The model under review builds one solid part; all positions refer to its coordinate system, in mm. Coordinates: 2 decimals unless noted, no trailing zeros. Write each loop counter-clockwise with the first axis right and the second up, starting at its lowest first coordinate (ties: lowest second). Pieces come first, ordered by that corner, then holes. Notation, with made-up numbers: (39.25, 48.5) - (47.25, 48.5) arc R14 cw to (47.25, 72.5) - close; hole circle Ø6 at (46.5, 87.5). An arc over 180 degrees is marked (long way). Put each result on its own line as item: value. Start each with the question number.
Item 1: To check wall thickness, follow L1, parallel to X at y = 3.5, z = -1; L2, parallel to X at y = 0.75, z = 25.5; L3, parallel to Z at x = 31, y = 3.5. State the ranges of each line that lie inside material, in increasing order. Write a range as [from, to].
Item 2: Consider section B-B on x = 0. Give the boundary of the cut face in (y, z), then the cut area to 3 significant figures.
Item 3: Consider section D-D on x = -56. Give the boundary of the cut face in (y, z).
Item 4: Consider section A-A on z = 0. Give the boundary of the cut face in (x, y), then the cut area to 3 significant figures.
Item 5: For pin 1 (1.9 mm diameter, centred on x = -60, y = 4.5, fed in from -Z); pin 2 (1.5 mm diameter, centred on y = 5.5, z = 41, fed in from +X); pin 3 (2 mm diameter, centred on y = 1, z = 42.5, fed in from +X), all flat-tipped, find the tip position at first contact; note any pin that passes through.
Item 6: Consider section C-C on z = 55. Give the boundary of the cut face in (x, y), then the cut area to 3 significant figures.
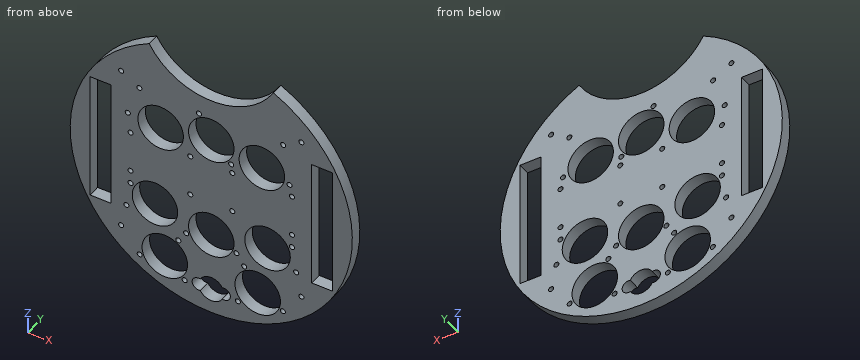
```python
from build123d import *

# Parameters (mm, degrees)
SKETCH1_R           = 1.35
SKETCH1_R_2         = 12.095
SKETCH1_W           = 11
SKETCH1_H           = 69
BOSS_EXTRUDE2_DEPTH = 6.35


with BuildPart() as part:
    # Sketch1 → Boss-Extrude2 (new body)
    with BuildSketch(Plane(origin=(0, 0, 0), x_dir=(1, 0, 0), z_dir=(0, 1, 0))):
        with BuildLine():
            ThreePointArc((32.995567884, -67.352004425), (0, 75), (-32.995567884, -67.352004425))
            ThreePointArc((-32.995567884, -67.352004425), (0, -48.302004425), (32.995567884, -67.352004425))
        make_face()
        with Locations((-42.910067426, 11.1)):
            Circle(SKETCH1_R, mode=Mode.SUBTRACT)
        with Locations((-42.910067426, -11.1)):
            Circle(SKETCH1_R, mode=Mode.SUBTRACT)
        with Locations((-11.160067426, -11.1)):
            Circle(SKETCH1_R, mode=Mode.SUBTRACT)
        with Locations((-11.160067426, 11.1)):
            Circle(SKETCH1_R, mode=Mode.SUBTRACT)
        with Locations((11.160067426, 11.1)):
            Circle(SKETCH1_R, mode=Mode.SUBTRACT)
        with Locations((11.160067426, -11.1)):
            Circle(SKETCH1_R, mode=Mode.SUBTRACT)
        with Locations((42.910067426, -11.1)):
            Circle(SKETCH1_R, mode=Mode.SUBTRACT)
        with Locations((42.910067426, 11.1)):
            Circle(SKETCH1_R, mode=Mode.SUBTRACT)
        with Locations((26.905821676, -20.904643604)):
            Circle(SKETCH1_R_2, mode=Mode.SUBTRACT)
        with Locations((24.699796409, 52.876021886)):
            Circle(SKETCH1_R_2, mode=Mode.SUBTRACT)
        with Locations((0, 29.793589551)):
            Circle(SKETCH1_R_2, mode=Mode.SUBTRACT)
        with Locations((0, -25.409190322)):
            Circle(SKETCH1_R_2, mode=Mode.SUBTRACT)
        with Locations((29.939937248, 24.651901309)):
            Circle(SKETCH1_R_2, mode=Mode.SUBTRACT)
        with Locations((-26.905821676, -20.904643604)):
            Circle(SKETCH1_R_2, mode=Mode.SUBTRACT)
        with Locations((-29.939937248, 24.651901309)):
            Circle(SKETCH1_R_2, mode=Mode.SUBTRACT)
        with Locations((17.503855967, 40.613487823)):
            Circle(SKETCH1_R, mode=Mode.SUBTRACT)
        with Locations((14.136463763, 62.392707439)):
            Circle(SKETCH1_R, mode=Mode.SUBTRACT)
        with Locations((38.046670289, 57.776252301)):
            Circle(SKETCH1_R, mode=Mode.SUBTRACT)
        with Locations((-42.910067426, 18.234848025)):
            Circle(SKETCH1_R, mode=Mode.SUBTRACT)
        with Locations((42.910067426, 18.234848025)):
            Circle(SKETCH1_R, mode=Mode.SUBTRACT)
        with Locations((-24.699796409, 52.876021886)):
            Circle(SKETCH1_R_2, mode=Mode.SUBTRACT)
        with Locations((45.13872464, 31.997163897)):
            Circle(SKETCH1_R, mode=Mode.SUBTRACT)
        with Locations((-45.13872464, 31.997163897)):
            Circle(SKETCH1_R, mode=Mode.SUBTRACT)
        with Locations((13.346873881, 34.693819966)):
            Circle(SKETCH1_R, mode=Mode.SUBTRACT)
        with Locations((-6.55476095, -38.026099982)):
            Circle(SKETCH1_R, mode=Mode.SUBTRACT)
        with Locations((-13.346873881, 34.693819966)):
            Circle(SKETCH1_R, mode=Mode.SUBTRACT)
        with Locations((10.597026674, -15.930038136)):
            Circle(SKETCH1_R, mode=Mode.SUBTRACT)
        with Locations((-38.234289702, -39.23697625)):
            Circle(SKETCH1_R, mode=Mode.SUBTRACT)
        with Locations((-47.92720717, -45.01204963)):
            Circle(SKETCH1_R, mode=Mode.SUBTRACT)
        with Locations((-47.92720717, 45.01204963)):
            Circle(SKETCH1_R, mode=Mode.SUBTRACT)
        with Locations((47.92720717, -45.01204963)):
            Circle(SKETCH1_R, mode=Mode.SUBTRACT)
        with Locations((-38.046670289, 57.776252301)):
            Circle(SKETCH1_R, mode=Mode.SUBTRACT)
        with Locations((-14.136463763, 62.392707439)):
            Circle(SKETCH1_R, mode=Mode.SUBTRACT)
        with Locations((-17.503855967, 40.613487823)):
            Circle(SKETCH1_R, mode=Mode.SUBTRACT)
        with Locations((47.92720717, 45.01204963)):
            Circle(SKETCH1_R, mode=Mode.SUBTRACT)
        with Locations((-44.385223141, -22.074211772)):
            Circle(SKETCH1_R, mode=Mode.SUBTRACT)
        with Locations((41.601681906, -17.457756634)):
            Circle(SKETCH1_R, mode=Mode.SUBTRACT)
        with Locations((38.234289702, -39.23697625)):
            Circle(SKETCH1_R, mode=Mode.SUBTRACT)
        with Locations((58.910067426, 0.102907352)):
            Rectangle(SKETCH1_W, SKETCH1_H, mode=Mode.SUBTRACT)
        with Locations((-58.910067426, 0.102907352)):
            Rectangle(SKETCH1_W, SKETCH1_H, mode=Mode.SUBTRACT)
        with BuildLine():
            ThreePointArc((-5.853899988, 64.744946271), (0.003726822, 68.153564176), (5.857575472, 64.738461857))
            ThreePointArc((5.857575472, 64.738461857), (10.16, 61.422565207), (5.857575472, 58.106668557))
            ThreePointArc((5.857575472, 58.106668557), (0.003726822, 54.691566239), (-5.853899988, 58.100184144))
            ThreePointArc((-5.853899988, 58.100184144), (-10.167207264, 61.422565207), (-5.853899988, 64.744946271))
        make_face(mode=Mode.SUBTRACT)
    extrude(amount=BOSS_EXTRUDE2_DEPTH)


solid = part.part
```
Report:
1. L1: [-74.99, -64.41], [-53.41, 53.41], [64.41, 74.99]
1. L2: [-70.53, -64.41], [-53.41, -38.09], [-15.72, -12.09], [12.09, 15.72], [38.09, 53.41], [64.41, 70.53]
1. L3: [-68.29, -63.2], [-42.55, -36.7], [-12.6, 9.52], [32.29, 64.25]
2. outline: (0, -75) - (6.35, -75) - (6.35, -68.15) - (0, -68.15) - close; (0, -54.69) - (6.35, -54.69) - (6.35, -41.89) - (0, -41.89) - close; (0, -17.7) - (6.35, -17.7) - (6.35, 13.31) - (0, 13.31) - close; (0, 37.5) - (6.35, 37.5) - (6.35, 48.3) - (0, 48.3) - close
2. area: 390 mm²
3. outline: (0, -49.89) - (6.35, -49.89) - (6.35, -34.6) - (0, -34.6) - close; (0, 34.4) - (6.35, 34.4) - (6.35, 49.89) - (0, 49.89) - close
4. outline: (-75, 0) - (-64.41, 0) - (-64.41, 6.35) - (-75, 6.35) - close; (-53.41, 0) - (53.41, 0) - (53.41, 6.35) - (-53.41, 6.35) - close; (64.41, 0) - (75, 0) - (75, 6.35) - (64.41, 6.35) - close
4. area: 813 mm²
5. pin 1: z = -46.24
5. pin 2: x = 63.28
5. pin 3: x = 62.47
6. outline: (-50.99, 0) - (-21.58, 0) - (-21.58, 6.35) - (-50.99, 6.35) - close; (21.58, 0) - (50.99, 0) - (50.99, 6.35) - (21.58, 6.35) - close
6. area: 374 mm²
